Here's how the part is built. I have some questions about the finished solid (model axes, mm). Face numbers are marked on the shaded views. A direction names the side the tool comes from. Round coordinates to 2 decimals unless told otherwise and drop trailing zeros. Loops run counter-clockwise (first coordinate to the right, second up) from the corner with the lowest first, then second, coordinate; pieces in that order, holes last. Notation, with made-up numbers: (34.5, 5) - (52.5, 5) arc R23 cw to (52.5, 38) - close; hole circle Ø8 at (51.25, 77). An arc over 180 degrees is marked (long way). Return JSON: item names as keys, results as strings. Group by question number.
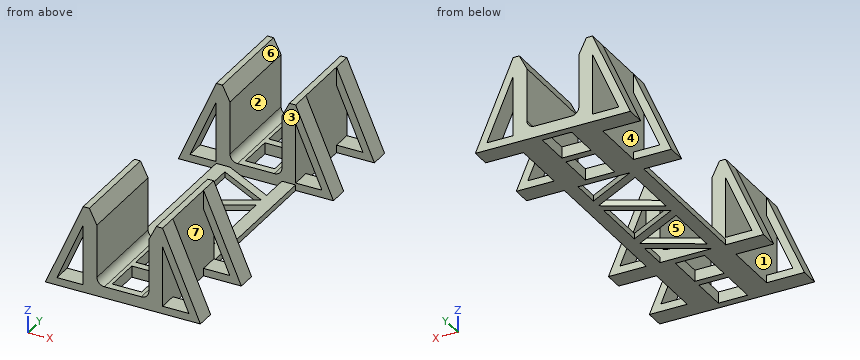
```python
from build123d import *

# Parameters (mm, degrees)
F1_DEPTH  = 114.3
F3_START  = 101.6
F3_DEPTH  = 12.7
F4_START  = 50.8
F4_DEPTH  = 12.7
F6_START  = 3.81
F5_W      = 53.34
F5_H      = 50.8
F6_DEPTH  = 54.61
F8_DEPTH  = 3.81
F9_R      = 5.08
F10_SIZE2 = 10.16
F10_SIZE  = 5.08
F11_SIZE2 = 5.08
F11_SIZE  = 10.16
F12_W     = 19.685
F12_H     = 24.13
F13_DEPTH = 7.62


with BuildPart() as f1:
    # F0 (on Front) → F1 (new body)
    with BuildSketch(Plane.XZ):
        Polygon((0, 58.42), (0, 0), (53.34, 0), (53.34, 58.42), (44.1325, 58.42), (44.1325, 7.62), (26.67, 7.62), (9.2075, 7.62), (9.2075, 58.42), align=None)
    extrude(amount=F1_DEPTH)

    # F2 (on Front) → F3 (join)
    with BuildSketch(Plane.XZ.offset(F3_START)):
        Polygon((78.74, 0), (53.34, 58.42), (53.34, 45.6794248168), (70.9919238334, 5.08), (53.34, 5.08), (53.34, 0), align=None)
        Polygon((-25.4, 0), (0, 0), (0, 5.08), (-17.6519238334, 5.08), (0, 45.6794248168), (0, 58.42), align=None)
    extrude(amount=F3_DEPTH)

    # F2 (on Front) → F4 (join)
    with BuildSketch(Plane.XZ.offset(F4_START)):
        Polygon((78.74, 0), (53.34, 58.42), (53.34, 45.6794248168), (70.9919238334, 5.08), (53.34, 5.08), (53.34, 0), align=None)
        Polygon((-25.4, 0), (0, 0), (0, 5.08), (-17.6519238334, 5.08), (0, 45.6794248168), (0, 58.42), align=None)
    extrude(amount=F4_DEPTH)

    # F5 (on Top) → F6 (cut)
    with BuildSketch(Plane.XY.offset(F6_START)):
        with Locations((26.67, -25.4)):
            Rectangle(F5_W, F5_H)
    extrude(amount=F6_DEPTH, mode=Mode.SUBTRACT)

    # F7 (on face) → F8 (cut, through all)
    with BuildSketch(Plane.XY):
        Polygon((44.1325, -31.75), (9.2075, -50.8), (44.1325, -50.8), align=None)
        Polygon((44.1325, -25.4), (9.2075, -6.35), (9.2075, -44.45), align=None)
        Polygon((44.1325, 0), (9.2075, 0), (44.1325, -19.05), align=None)
    extrude(amount=F8_DEPTH, mode=Mode.SUBTRACT)

    # F9
    f9_edges = [f1.edges().sort_by_distance(p)[0] for p in [
        (9.2075, -82.55, 7.62),
        (44.1325, -82.55, 7.62),
    ]]
    fillet(f9_edges, radius=F9_R)

    # F10
    f10_edges = [f1.edges().sort_by_distance(p)[0] for p in [
        (9.2075, -82.55, 58.42),
    ]]
    f10_side = f1.faces().sort_by_distance((4.60375, -82.55, 58.42))[0]
    chamfer(f10_edges, length=F10_SIZE, length2=F10_SIZE2, reference=f10_side)

    # F11
    f11_edges = [f1.edges().sort_by_distance(p)[0] for p in [
        (44.1325, -82.55, 58.42),
    ]]
    f11_side = f1.faces().sort_by_distance((44.1325, -82.55, 35.56))[0]
    chamfer(f11_edges, length=F11_SIZE, length2=F11_SIZE2, reference=f11_side)

    # F12 (on face) → F13 (cut, through all)
    with BuildSketch(Plane.XY.offset(7.62)):
        with Locations((26.67, -67.945)):
            Rectangle(F12_W, F12_H)
        with Locations((26.67, -97.155)):
            Rectangle(F12_W, F12_H)
    extrude(amount=-F13_DEPTH, mode=Mode.SUBTRACT)

    # F14: F1 across plane


with BuildPart() as f1_1:
    add(f1.part)
    add(f1.part.mirror(Plane.XZ))


solid = f1_1.part
```
Q1. Imagine slicing it at C-C, the plane y = -35. List the corners of the cut face in (x, z) for me, and give its area (3 significant figures).
Q2. For the marked faces 1, 2 and 3, which set-ups out of +Z, -Z, +X, -X, +Y, -Y let a thin tool reach every point of the face, with its end or its side?
Q3. Imagine slicing it at A-A, the plane y = -69.5. List the corners of the cut face in (x, z) for me.
Q4. Imagine slicing it at D-D, the plane x = 12. List the corners of the cut face in (y, z) for me, and give its area (3 significant figures).
Q5. If we mould it in two halves opening along Z, with no side actions, what happens to the marked faces 4, 5, 6 and 7? For each: +Z half, -Z half, draft (parallel to the pull), parting line (faces both ways), or undercut.
Q6. Please list where these lines run through material, in increasing order: line 1 (Y direction, x = 65, z = 26); line 2 (Y direction, x = 32.5, z = 5.5); line 3 (X direction, y = 74, z = 28.5).
Q7. Will these pins go through, and if not, where does the flat tip stop? pin 1 Ø4 at (x, y) = (-6.5, -57) entering from +Z; pin 2 Ø4 at (y, z) = (-69.5, 2) entering from +X; pin 3 Ø2.5 at (y, z) = (-97.5, 5) entering from -X; pin 4 Ø4 at (x, z) = (67.5, 31) entering from -Y.
Q8. Imagine slicing it at B-B, the plane x = -5. Give the number of separate pieces and of enclosed holes in the cut face, and give its area (3 significant figures).
Output values:
{
 "1": {"outline": "(0, 0) - (9.21, 0) - (9.21, 3.81) - (0, 3.81) - close; (26.53, 0) - (38.17, 0) - (38.17, 3.81) - (26.53, 3.81) - close; (44.13, 0) - (53.34, 0) - (53.34, 3.81) - (44.13, 3.81) - close", "area": "115 mm^2"},
 "2": {"face 1": "none", "face 2": "+Z, +Y, -Y", "face 3": "+Z"},
 "3": {"outline": "(0, 0) - (16.83, 0) - (16.83, 7.62) - (14.29, 7.62) arc R5.08 cw to (9.21, 12.7) - (9.21, 48.26) - (4.13, 58.42) - (0, 58.42) - close; (36.51, 0) - (53.34, 0) - (53.34, 58.42) - (49.21, 58.42) - (44.13, 48.26) - (44.13, 12.7) arc R5.08 cw to (39.05, 7.62) - (36.51, 7.62) - close"},
 "4": {"outline": "(-114.3, 0) - (-50.8, 0) - (-50.8, 8.16) - (-114.3, 8.16) - close; (-49.28, 0) - (-42.93, 0) - (-42.93, 3.81) - (-49.28, 3.81) - close; (-7.87, 0) - (-1.52, 0) - (-1.52, 3.81) - (-7.87, 3.81) - close; (1.52, 0) - (7.87, 0) - (7.87, 3.81) - (1.52, 3.81) - close; (42.93, 0) - (49.28, 0) - (49.28, 3.81) - (42.93, 3.81) - close; (50.8, 0) - (114.3, 0) - (114.3, 8.16) - (50.8, 8.16) - close", "area": "1,130 mm^2"},
 "5": {"face 4": "undercut", "face 5": "draft", "face 6": "+Z half", "face 7": "undercut"},
 "6": {"line 1": "y = -114.3 to -101.6, -63.5 to -50.8, 50.8 to 63.5, 101.6 to 114.3", "line 2": "y = -114.3 to -109.22, -85.09 to -80.01, -55.88 to -50.8, 50.8 to 55.88, 80.01 to 85.09, 109.22 to 114.3", "line 3": "x = 0 to 9.21, 44.13 to 53.34"},
 "7": {"pin 1": "stops at z = 48.07", "pin 2": "stops at x = 53.34", "pin 3": "stops at x = 0", "pin 4": "passes through"},
 "8": {"separate pieces": "8", "enclosed holes": "0", "area": "905 mm^2"}
}
